Could you check a few things on this model? Use its own coordinates, in mm. Face numbers are marked on the shaded views. Give positions to 0.01 mm unless a question says otherwise; leave off trailing zeros. Order: outer loops, then holes, each group sorted by start corner. A loop starts at its lowest first (then second) coordinate and runs counter-clockwise, first axis right, second up. Notation, with made-up numbers: (71, 9.5) - (78, 9.5) arc R11 ccw to (78, 15.5) - close; hole circle Ø11 at (-1.75, -24.75). An arc over 180 degrees is marked (long way). Put each result on its own line as item: value.
from build123d import *

# Parameters (mm, degrees)
F0_R     = 32.5
F1_DEPTH = 3


with BuildPart() as f1:
    # F0 (on Right) → F1 (new body)
    with BuildSketch(Plane.YZ):
        with BuildLine():
            ThreePointArc((90, 54.586), (88.535534, 58.121534), (85, 59.586))
            Line((85, 59.586), (40, 59.586))
            Line((40, 59.586), (40, 54.586))
            Line((40, 54.586), (40, 45.586))
            Line((40, 45.586), (-40, 45.586))
            Line((-40, 45.586), (-40, 54.586))
            Line((-40, 54.586), (-40, 59.586))
            Line((-40, 59.586), (-85, 59.586))
            ThreePointArc((-85, 59.586), (-88.535534, 58.121534), (-90, 54.586))
            Line((-90, 54.586), (-90, -35.414))
            ThreePointArc((-90, -35.414), (-88.535534, -38.949534), (-85, -40.414))
            Line((-85, -40.414), (85, -40.414))
            ThreePointArc((85, -40.414), (88.535534, -38.949534), (90, -35.414))
            Line((90, -35.414), (90, 54.586))
        make_face()
        Circle(F0_R, mode=Mode.SUBTRACT)
    extrude(amount=F1_DEPTH)


solid = f1.part
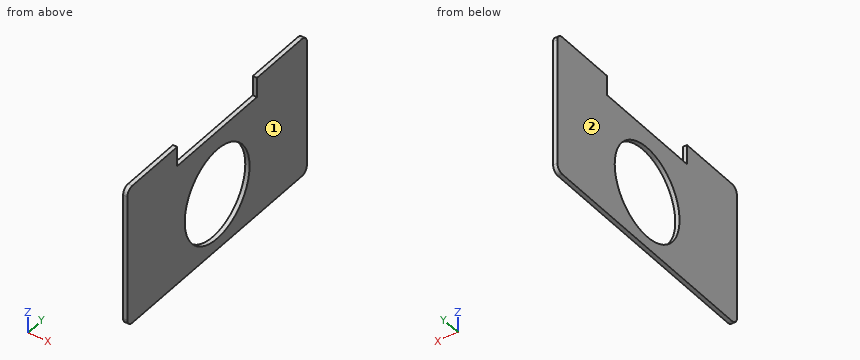
1) I'm going to push a flat-ended pin straight in: pin 1 (1.5 mm diameter, centred on x = 1.5, y = 2.5, fed in from +Z). Where does the tip first touch, or does it pass through?
Filled in:
pin 1: stops at z = 45.59
2) Suppose I cut it at C-C, the plane x = 1.6. List the corners of the cut face in (y, z) for me, and give its area (3 significant figures).
Filled in:
outline: (-90, -35.41) arc R5 ccw to (-85, -40.41) - (85, -40.41) arc R5 ccw to (90, -35.41) - (90, 54.59) arc R5 ccw to (85, 59.59) - (40, 59.59) - (40, 45.59) - (-40, 45.59) - (-40, 59.59) - (-85, 59.59) arc R5 ccw to (-90, 54.59) - close; hole circle Ø65 at (0, 0)
area: 13,500 mm^2
3) Suppose I cut it at A-A, the plane z = 0. List the corners of the cut face in (x, y) for me, and give its area (3 significant figures).
Filled in:
outline: (0, -90) - (3, -90) - (3, -32.5) - (0, -32.5) - close; (0, 32.5) - (3, 32.5) - (3, 90) - (0, 90) - close
area: 345 mm^2
4) We'd pull the mould along X, two halves only. Please class the marked faces 1 and 2: pulls with the +X half, pulls with the -X half, needs draft (parallel to the pull), parting line crosses it, or undercut.
Filled in:
face 1: pulls with the +X half
face 2: pulls with the -X half
5) Suppose I cut it at B-B, the plane y = 0. List the corners of the cut face in (x, z) for me.
Filled in:
outline: (0, -40.41) - (3, -40.41) - (3, -32.5) - (0, -32.5) - close; (0, 32.5) - (3, 32.5) - (3, 45.59) - (0, 45.59) - close
6) If I drill on line 1 (Z direction, x = 0.8, y = 0); line 2 (Y direction, x = 1.65, z = -24.5); line 3 (Y direction, x = 1.8, z = 10), over which ranges is the centre line in solid material (lowest first)? Write a range as [from, to].
Filled in:
line 1: z = [-40.41, -32.5], [32.5, 45.59]
line 2: y = [-90, -21.35], [21.35, 90]
line 3: y = [-90, -30.92], [30.92, 90]
